Could you check a few things on this model? Use its own coordinates, in mm. Face numbers are marked on the shaded views. A direction names the side the tool comes from. Round coordinates to 2 decimals unless told otherwise and drop trailing zeros. Write each loop counter-clockwise with the first axis right and the second up, starting at its lowest first coordinate (ties: lowest second). Pieces come first, ordered by that corner, then holes. Notation, with made-up numbers: (-9.5, 16.5) -> (6.5, 16.5) arc R28 cw to (6.5, 50.5) -> close; hole circle Ø6 at (41, -15). An arc over 180 degrees is marked (long way). Answer in a Markdown table with one row per item.
from build123d import *

# Parameters (mm, degrees)
BOSS_EXTRUDE1_DEPTH = 12.15
SKETCH4_R           = 1
CUT_EXTRUDE1_DEPTH  = 12.15
SKETCH5_R           = 6
SKETCH5_R_2         = 3
BOSS_EXTRUDE2_DEPTH = 5
SKETCH6_R           = 2
BOSS_EXTRUDE3_DEPTH = 2
SKETCH7_R           = 3.615
BOSS_EXTRUDE4_DEPTH = 6
BOSS_EXTRUDE5_START = -2.79
BOSS_EXTRUDE5_DEPTH = 2


with BuildPart() as part:
    # Sketch3 → Boss-Extrude1 (new body)
    with BuildSketch(Plane.XY):
        Polygon((8.87359736, -19.274521452), (-14.12640264, -19.274521452), (-14.12640264, -0.664521452), (-18.62640264, -0.664521452), (-18.62640264, 1.535478548), (-14.12640264, 1.535478548), (-14.12640264, 3.535478548), (8.87359736, 3.535478548), (8.87359736, 1.535478548), (13.37359736, 1.535478548), (13.37359736, -0.664521452), (8.87359736, -0.664521452), align=None)
    extrude(amount=BOSS_EXTRUDE1_DEPTH)

    # Sketch4 → Cut-Extrude1 (cut)
    with BuildSketch(Plane(origin=(0, 1.535478548, 0), x_dir=(1, 0, 0), z_dir=(0, 1, 0))):
        with Locations(Location((-16.62640264, -6.075, 0), (0, 0, 270))):
            Circle(SKETCH4_R)
        with Locations(Location((11.37359736, -6.075, 0), (0, 0, 270))):
            Circle(SKETCH4_R)
    extrude(amount=-CUT_EXTRUDE1_DEPTH, mode=Mode.SUBTRACT)

    # Sketch5 → Boss-Extrude2 (add)
    with BuildSketch(Plane(origin=(0, 3.535478548, 0), x_dir=(1, 0, 0), z_dir=(0, 1, 0))):
        with Locations((-8.12640264, -6.075)):
            Circle(SKETCH5_R)
        with Locations((-2.12640264, -6.075)):
            Circle(SKETCH5_R_2)
    extrude(amount=BOSS_EXTRUDE2_DEPTH)

    # Sketch6 → Boss-Extrude3 (add)
    with BuildSketch(Plane(origin=(0, 8.535478548, 0), x_dir=(1, 0, 0), z_dir=(0, 1, 0))):
        with Locations(Location((-8.12640264, -6.075, 0), (0, 0, 270))):
            Circle(SKETCH6_R)
    extrude(amount=BOSS_EXTRUDE3_DEPTH)

    # Sketch7 → Boss-Extrude4 (add)
    with BuildSketch(Plane(origin=(0, 10.535478548, 0), x_dir=(1, 0, 0), z_dir=(0, 1, 0))):
        with Locations(Location((-8.12640264, -6.075, 0), (0, 0, 270))):
            Circle(SKETCH7_R)
    extrude(amount=BOSS_EXTRUDE4_DEPTH)

    # Sketch8 → Boss-Extrude5 (add)
    with BuildSketch(Plane(origin=(0, 16.535478548, 0), x_dir=(1, 0, 0), z_dir=(0, 1, 0)).offset(BOSS_EXTRUDE5_START)):
        with BuildLine():
            ThreePointArc((-7.720547583, -2.482854865), (-5.430536264, -3.666571159), (-4.51140264, -6.075))
            Line((-4.51140264, -6.075), (4.25859736, -6.075))
            ThreePointArc((4.25859736, -6.075), (4.92613327, -4.583510995), (6.483136811, -4.087644462))
            Line((6.483136811, -4.087644462), (-7.720547583, -2.482854865))
        make_face()
        with BuildLine():
            Line((4.25859736, -6.075), (-4.51140264, -6.075))
            ThreePointArc((-4.51140264, -6.075), (-5.430536264, -8.483428841), (-7.720547583, -9.667145135))
            Line((-7.720547583, -9.667145135), (6.483136811, -8.062355538))
            ThreePointArc((6.483136811, -8.062355538), (4.92613327, -7.566489005), (4.25859736, -6.075))
        make_face()
        with BuildLine():
            ThreePointArc((6.483136811, -4.087644462), (4.92613327, -4.583510995), (4.25859736, -6.075))
            Line((4.25859736, -6.075), (8.25859736, -6.075))
            ThreePointArc((8.25859736, -6.075), (7.750086364, -4.742535911), (6.483136811, -4.087644462))
        make_face()
        with BuildLine():
            Line((8.25859736, -6.075), (4.25859736, -6.075))
            ThreePointArc((4.25859736, -6.075), (4.92613327, -7.566489005), (6.483136811, -8.062355538))
            ThreePointArc((6.483136811, -8.062355538), (7.750086364, -7.407464089), (8.25859736, -6.075))
        make_face()
    extrude(amount=BOSS_EXTRUDE5_DEPTH)


solid = part.part
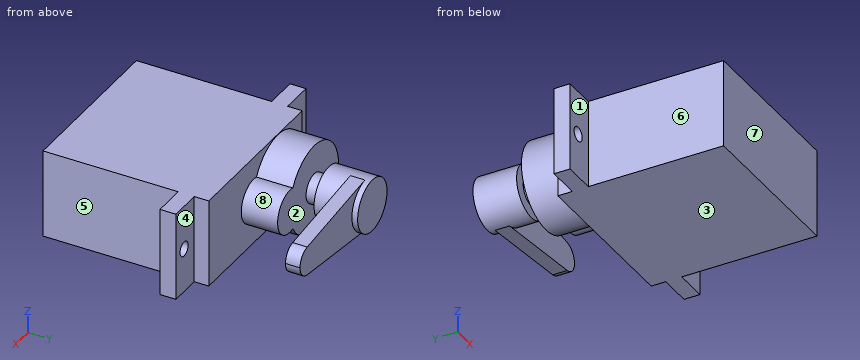
1) Imagine slicing it at B-B, the plane x = 6. Please give me the cut outline in (y, z).
Findings:
| item | result |
|---|---|
| outline | (-19.27, 0) -> (3.54, 0) -> (3.54, 12.15) -> (-19.27, 12.15) -> close; (13.75, 4.03) -> (15.75, 4.03) -> (15.75, 8.12) -> (13.75, 8.12) -> close |
2) For pin 1 (3.5 mm diameter, centred on y = -8.5, z = 7, fed in from +X); pin 2 (1.3 mm diameter, centred on x = -16.5, z = 6.5, fed in from -Y); pin 3 (1 mm diameter, centred on y = 2.5, z = 8.5, fed in from -X); pin 4 (1.8 mm diameter, centred on x = 11.37, z = 6.08, fed in from +Y), each with a flat end and sliding along its axis, tell me the tip position at first contact or that it passes through.
Findings:
| item | result |
|---|---|
| pin 1 | stops at x = 8.87 |
| pin 2 | stops at y = -0.66 |
| pin 3 | stops at x = -14.13 |
| pin 4 | passes through |
3) Imagine slicing it at C-C, the plane y = 0. Please give me the cut outline in (x, z) (3 decimals), plus the area to 3 significant figures.
Findings:
| item | result |
|---|---|
| outline | (-18.626, 0) -> (13.374, 0) -> (13.374, 12.15) -> (-18.626, 12.15) -> close; hole circle Ø2 at (-16.626, 6.075); hole circle Ø2 at (11.374, 6.075) |
| area | 383 mm^2 |
4) Thinking about a two-plate mould opening in X: for the marked faces 6, 7 and 8, which applies, +X half, -X half, draft (parallel to the pull), parting line (faces both ways), or undercut?
Findings:
| item | result |
|---|---|
| face 6 | -X half |
| face 7 | draft |
| face 8 | undercut |
5) Please list where these lines run through material, in increasing order: line 1 (Y direction, x = -6, z = 7.5); line 2 (Y direction, x = 7.5, z = 6.5); line 3 (X direction, y = -6.5, z = 6.5).
Findings:
| item | result |
|---|---|
| line 1 | y = -19.27 to 8.54, 10.54 to 16.54 |
| line 2 | y = -19.27 to 3.54, 13.75 to 15.75 |
| line 3 | x = -14.13 to 8.87 |
6) For the marked faces 1, 2, 3, 4 and 5, which set-ups out of +Z, -Z, +X, -X, +Y, -Y let a thin tool reach every point of the face, with its end or its side?
Findings:
| item | result |
|---|---|
| face 1 | +Z, -Z, -X, -Y |
| face 2 | none |
| face 3 | -Z, +X, -X, +Y, -Y |
| face 4 | +Z, -Z, +X, +Y |
| face 5 | +Z, -Z, +X, -Y |
7) Imagine slicing it at A-A, the plane z = 8.5. Please give me the cut outline in (x, y).
Findings:
| item | result |
|---|---|
| outline | (-18.63, -0.66) -> (-14.13, -0.66) -> (-14.13, -19.27) -> (8.87, -19.27) -> (8.87, -0.66) -> (13.37, -0.66) -> (13.37, 1.54) -> (8.87, 1.54) -> (8.87, 3.54) -> (-0.36, 3.54) -> (-0.36, 8.54) -> (-13.61, 8.54) -> (-13.61, 3.54) -> (-14.13, 3.54) -> (-14.13, 1.54) -> (-18.63, 1.54) -> close; (-10.81, 10.54) -> (-5.45, 10.54) -> (-5.45, 13.75) -> (2.61, 13.75) -> (2.61, 15.75) -> (-5.45, 15.75) -> (-5.45, 16.54) -> (-10.81, 16.54) -> close |
8) Imagine slicing it at D-D, the plane y = -14. Please give me the cut outline in (x, z), plus the area to 3 significant figures.
Findings:
| item | result |
|---|---|
| outline | (-14.13, 0) -> (8.87, 0) -> (8.87, 12.15) -> (-14.13, 12.15) -> close |
| area | 279 mm^2 |
